Here's how the part is built. I have some questions about the finished solid (model axes, mm). A direction names the side the tool comes from. Coordinates: 2 decimals unless noted, no trailing zeros. Write each loop counter-clockwise with the first axis right and the second up, starting at its lowest first coordinate (ties: lowest second). Pieces come first, ordered by that corner, then holes.
(1) Please list where these lines run through material, in increasing order: probe 1 along Y at (x, z) = (10, -37.7); probe 2 along X at (y, z) = (15.75, 107.5); probe 3 along Y at (x, z) = (10, -36.75).
(2) Thinking about a two-plate mould opening in Z: for faces 4 (the cylindrical face through (9.912, 20.248, 143.786)), 5 (the cylindrical face through (2.85, -5.22, -37.68)), 6 (the cylindrical face through (9.912, 20.248, 73.786)), 7 (the flat face through (5, 9, -35.213)), which applies, released by +Z, released by -Z, zero draft, split by the parting line, or undercut?
(3) Which directions (+Z, -Z, +X, -X, +Y, -Y) give clear straight access to the entire face, cutting with the end or side of a thin tool? Please do faces 1 (the cylindrical face through (10.09, 20.25, 60.79)), 2 (the flat face through (5.7, 18.769, 65.1)), 3 (the flat face through (0, 16, 57)).
(4) Imagine slicing it at A-A, the plane z = 54. List the corners of the cut face in (x, y) for me, plus the area to 3 significant figures.
(5) For pin 1 Ø10 at (x, z) = (9, 27) entering from -Y; pin 2 Ø0.8 at (x, z) = (1.5, 68) entering from -Y; pin 3 Ø8 at (x, y) = (14, 5) entering from -Z; pin 4 Ø11.5 at (x, y) = (10, 1.77) entering from -Z, each with a flat end and sliding along its axis, tell me the tip position at first contact or that it passes through.
```python
from build123d import *

# Parameters (mm, degrees)
BOSS_EXTRUDE1_DEPTH = 20
CUT_EXTRUDE1_DEPTH  = 20
LPATTERN1_COUNT     = 2
LPATTERN1_PITCH     = 70
SKETCH3_R           = 6.5
CUT_EXTRUDE2_DEPTH  = 20
FILLET1_R           = 3
FILLET2_R           = 10
CHAMFER1_SIZE       = 1
FILLET3_R           = 3
SKETCH4_W           = 2.5
SKETCH4_H           = 193.282741961
BOSS_EXTRUDE2_DEPTH = 7
LPATTERN2_COUNT     = 2
LPATTERN2_PITCH     = 17.5
CHAMFER2_SIZE       = 27.474774195
CHAMFER2_SIZE_2     = 10
FILLET4_R           = 10
FILLET5_R           = 2


# Some blends are built 0.0001 mm under size
with BuildPart() as part:
    # Sketch1 → Boss-Extrude1 (new body)
    with BuildSketch(Plane(origin=(0, 0, 0), x_dir=(0, 0, -1), z_dir=(1, 0, 0))):
        Polygon((-159.787234043, 21.769316909), (40.212765957, 21.769316909), (40.212765957, -8.230683091), (35.212765957, -8.230683091), (35.212765957, 18.769316909), (-159.787234043, 18.769316909), align=None)
    extrude(amount=BOSS_EXTRUDE1_DEPTH)

    # Sketch2 → Cut-Extrude1 (cut)
    with BuildSketch(Plane.XZ.offset(-18.769316909)):
        with BuildLine():
            Line((14, 139.787234043), (14, 134.787234043))
            ThreePointArc((14, 134.787234043), (10, 130.787234043), (6, 134.787234043))
            Line((6, 134.787234043), (6, 139.787234043))
            ThreePointArc((6, 139.787234043), (10, 143.787234043), (14, 139.787234043))
        make_face()
    cut_extrude1 = extrude(amount=-CUT_EXTRUDE1_DEPTH, mode=Mode.SUBTRACT)

    # LPattern1: Cut-Extrude1 ×2
    with Locations(*[(0, 0, -i * LPATTERN1_PITCH) for i in range(1, LPATTERN1_COUNT)]):
        add(cut_extrude1, mode=Mode.SUBTRACT)

    # Sketch3 → Cut-Extrude2 (cut)
    with BuildSketch(Plane.XY.offset(-35.212765957)):
        with Locations((10, 1.769316909)):
            Circle(SKETCH3_R)
    extrude(amount=-CUT_EXTRUDE2_DEPTH, mode=Mode.SUBTRACT)

    # Fillet1
    fillet1_edges = [part.edges().sort_by_distance(p)[0] for p in [
        (10, 21.769316909, -40.212765957),
        (10, 18.769316909, -35.212765957),
    ]]
    fillet(fillet1_edges, radius=FILLET1_R)

    # Fillet2
    fillet2_edges = [part.edges().sort_by_distance(p)[0] for p in [
        (0, -8.230683091, -37.712765957),
        (20, -8.230683091, -37.712765957),
    ]]
    fillet(fillet2_edges, radius=FILLET2_R - 0.0001)  # a hair under: the kernel refuses the full size

    # Chamfer1
    chamfer1_edges = [part.edges().sort_by_distance(p)[0] for p in [
        (3.5, 1.769316909, -40.212765957),
        (3.5, 1.769316909, -35.212765957),
    ]]
    chamfer(chamfer1_edges, length=CHAMFER1_SIZE)

    # Fillet3
    fillet3_edges = [part.edges().sort_by_distance(p)[0] for p in [
        (20, 20.269316909, 159.787234043),
        (0, 20.269316909, 159.787234043),
    ]]
    fillet(fillet3_edges, radius=FILLET3_R)

    # Sketch4 → Boss-Extrude2 (add)
    with BuildSketch(Plane.XZ.offset(-18.769316909)):
        with Locations((1.25, 58.701442972)):
            Rectangle(SKETCH4_W, SKETCH4_H)
    boss_extrude2 = extrude(amount=BOSS_EXTRUDE2_DEPTH)

    # LPattern2: Boss-Extrude2 ×2
    with Locations(*[(i * LPATTERN2_PITCH, 0, 0) for i in range(1, LPATTERN2_COUNT)]):
        add(boss_extrude2)

    # Chamfer2
    # the kernel refuses this chamfer: 27.474774195, 10 mm, written as the material it takes off along each edge
    with BuildSketch(Plane(origin=(73.774914494, 11.769316909, 155.342813952), x_dir=(0, -0.013184058198645638, -0.9999130865277315), z_dir=(-1, 0, 0))) as chamfer2_piece_1_section:
        Polygon((CHAMFER2_SIZE * 0.999913086511, -CHAMFER2_SIZE * 0.0131840581984), (-CHAMFER2_SIZE_2 * 0.0131840581986, -CHAMFER2_SIZE_2 * 0.999913086528), (0, 0), align=None)
    chamfer2_piece_1 = extrude(amount=145.049828987, mode=Mode.PRIVATE)
    chamfer2_piece_1 = split(chamfer2_piece_1, bisect_by=Plane(origin=(1.25, 18.769316909, 145.126312786), z_dir=(0, -1, 0)), keep=Keep.TOP, mode=Mode.PRIVATE)
    add(chamfer2_piece_1, mode=Mode.SUBTRACT)
    with BuildSketch(Plane(origin=(91.274914494, 11.769316909, 155.342813952), x_dir=(0, -0.013184058198645638, -0.9999130865277315), z_dir=(-1, 0, 0))) as chamfer2_piece_2_section:
        Polygon((CHAMFER2_SIZE * 0.999913086511, -CHAMFER2_SIZE * 0.0131840581984), (-CHAMFER2_SIZE_2 * 0.0131840581986, -CHAMFER2_SIZE_2 * 0.999913086528), (0, 0), align=None)
    chamfer2_piece_2 = extrude(amount=145.049828987, mode=Mode.PRIVATE)
    chamfer2_piece_2 = split(chamfer2_piece_2, bisect_by=Plane(origin=(18.75, 18.769316909, 145.126312786), z_dir=(0, -1, 0)), keep=Keep.TOP, mode=Mode.PRIVATE)
    add(chamfer2_piece_2, mode=Mode.SUBTRACT)

    # Fillet4
    fillet4_edges = [part.edges().sort_by_distance(p)[0] for p in [
        (1.25, 11.769316909, 127.868039758),
        (18.75, 11.769316909, 127.868039758),
        (1.25, 18.769316909, 147.100381694),
        (18.75, 18.769316909, 147.100381694),
    ]]
    fillet(fillet4_edges, radius=FILLET4_R)

    # Fillet5
    fillet5_edges = [part.edges().sort_by_distance(p)[0] for p in [
        (1.25, 11.769316909, -35.212765957),
        (18.75, 11.769316909, -35.212765957),
    ]]
    fillet(fillet5_edges, radius=FILLET5_R)


solid = part.part
```
Recorded:
1. probe 1: y = -8.23 to -4.73, 8.27 to 21.73
1. probe 2: x = 0 to 2.5, 17.5 to 20
1. probe 3: y = -8.23 to -4.73, 8.27 to 21.77
2. face 4: undercut
2. face 5: zero draft
2. face 6: undercut
2. face 7: released by +Z
3. face 1: +Y, -Y
3. face 2: +Z, -Y
3. face 3: +Z, -Z, -X, +Y, -Y
4. outline: (0, 11.77) - (2.5, 11.77) - (2.5, 18.77) - (17.5, 18.77) - (17.5, 11.77) - (20, 11.77) - (20, 21.77) - (0, 21.77) - close
4. area: 95.0 mm2
5. pin 1: stops at y = 18.77
5. pin 2: stops at y = 11.77
5. pin 3: stops at z = -40.21
5. pin 4: passes through
